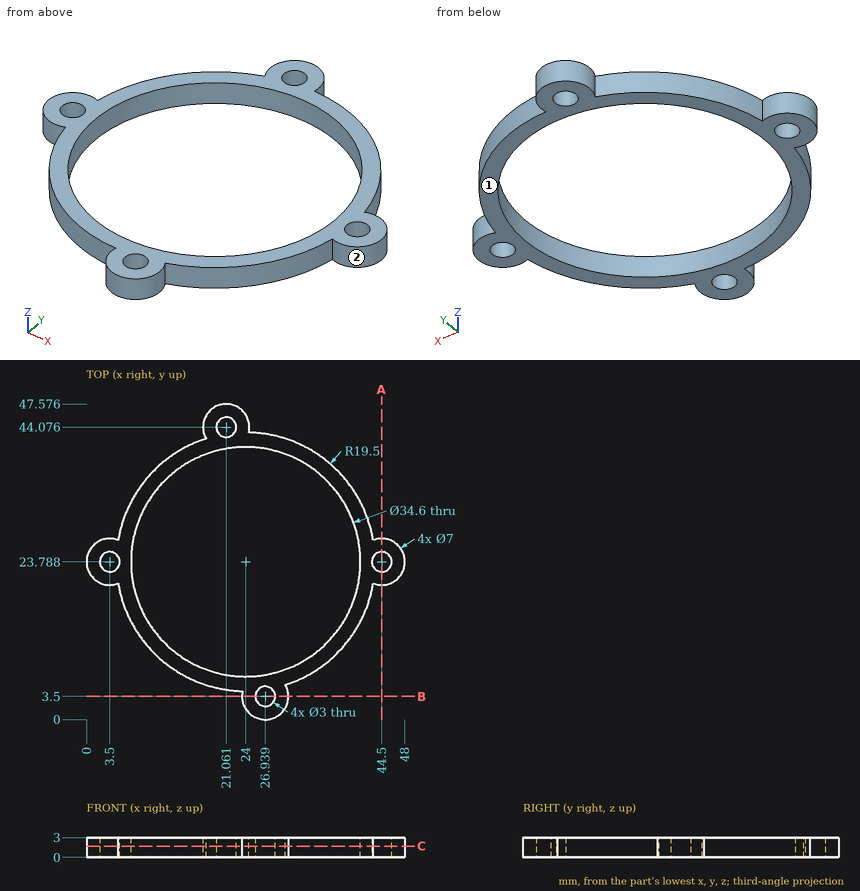
Check sheet for the drawn part. Datum: minimum x, y, z corner. Units: mm. Give positions to 0.01 mm unless a question says otherwise; leave off trailing zeros. Loops run counter-clockwise (first coordinate to the right, second up) from the corner with the lowest first, then second, coordinate; pieces in that order, holes last. Notation, with made-up numbers: (-38, 14) - (19, 14) arc R19 cw to (19, 27) - close; hole circle Ø6 at (42, -4). An arc over 180 degrees is marked (long way). Write each question's results on one line, items separated by ' | '.
1) Material ranges on L1, parallel to X at y = 25, z = 0.7 (1 decimal); L2, parallel to Y at x = 3.5, z = 0.7; L3, parallel to X at y = 10, z = 0.9, recorded low to high. Write a range as from..to.
Solution:
L1: 0.2..2.6, 4.4..6.7, 41.3..43.6, 45.4..47.8 | L2: 20.29..22.29, 25.29..27.29 | L3: 10.21..13.55, 34.45..37.79
2) Depth check by flat-ended pin: P1, Ø2.5, axis at x = 3.5, y = 23.79, coming from the +Z side. Enter the tip coordinate at first touch or a pass-through.
Solution:
P1: through
3) Sectioned sample at B-B on y = 3.5. Record the boundary of the cut face in (x, z), plus the area to 3 significant figures.
Solution:
outline: (23.44, 0) - (25.44, 0) - (25.44, 3) - (23.44, 3) - close; (28.44, 0) - (30.44, 0) - (30.44, 3) - (28.44, 3) - close | area: 12.0 mm2
4) Sectioned sample at A-A on x = 44.5. Record the boundary of the cut face in (y, z), plus the area to 3 significant figures.
Solution:
outline: (20.29, 0) - (22.29, 0) - (22.29, 3) - (20.29, 3) - close; (25.29, 0) - (27.29, 0) - (27.29, 3) - (25.29, 3) - close | area: 12.0 mm2
5) Sectioned sample at C-C on z = 1.7. Record the boundary of the cut face in (x, y) (1 decimal), plus the area to 3 significant figures.
Solution:
outline: (4.8, 20.5) arc R19.5 ccw to (23.5, 4.3) arc R3.5 ccw (long way) to (30, 5.2) arc R19.5 ccw to (43.2, 20.5) arc R3.5 ccw (long way) to (43.2, 27) arc R19.5 ccw to (24.5, 43.3) arc R3.5 ccw (long way) to (18, 42.3) arc R19.5 ccw to (4.8, 27) arc R3.5 ccw (long way) to start; hole circle Ø3 at (3.5, 23.8); hole circle Ø34.6 at (24, 23.8); hole circle Ø3 at (21.1, 44.1); hole circle Ø3 at (26.9, 3.5); hole circle Ø3 at (44.5, 23.8) | area: 333 mm2
6) Mould release check, pull along X, two halves, no side actions. Record for the marked faces 1 and 2: pulls with the +X half, pulls with the -X half, needs draft (parallel to the pull), parting line crosses it, or undercut.
Solution:
face 1: needs draft | face 2: undercut
